```python
from build123d import *

# Parameters (mm, degrees)
BOSS_EXTRUDE1_DEPTH = 3
FILLET1_R           = 10
FILLET2_R           = 2
FILLET3_R           = 4
FILLET4_R           = 1
FILLET5_R           = 2
FILLET6_R           = 3
FILLET7_R           = 2
FILLET8_R           = 1


with BuildPart() as part:
    # Sketch1 → Boss-Extrude1 (new body)
    with BuildSketch(Plane(origin=(0, 0, 0), x_dir=(1, 0, 0), z_dir=(0, 1, 0))):
        with BuildLine():
            Line((0, 0), (0, 7.21))
            ThreePointArc((0, 7.21), (1.5, 8.71), (3, 7.21))
            Line((3, 7.21), (3, 0))
            ThreePointArc((3, 0), (10.063508451, 2.530649612), (15.2, 8))
            Line((15.2, 8), (20.9, 10.15))
            Line((20.9, 10.15), (22, 15.56))
            Line((22, 15.56), (30.53, 20))
            Line((30.53, 20), (21.94, 28))
            Line((21.94, 28), (18.834507406, 25.494802254))
            Line((18.834507406, 25.494802254), (22.601722061, 20.824888578))
            Line((22.601722061, 20.824888578), (16.53, 18.68))
            ThreePointArc((16.53, 18.68), (13.852574152, 13.870404311), (8.467766761, 12.728183128))
            Line((8.467766761, 12.728183128), (-3.6, 15.4))
            Line((-3.6, 15.4), (-6, 24.68))
            Line((-6, 24.68), (-7.84518958, 28))
            Line((-7.84518958, 28), (-8.88, 34.5))
            Line((-8.88, 34.5), (-2.152236064, 35.529882091))
            Line((-2.152236064, 35.529882091), (-2.387170471, 36.974018228))
            ThreePointArc((-2.387170471, 36.974018228), (-7.295622624, 39.289989721), (-12.7222653, 39.199569746))
            Line((-12.7222653, 39.199569746), (-14.412236064, 37.968616292))
            Line((-14.412236064, 37.968616292), (-12.083283256, 30.98175787))
            Line((-12.083283256, 30.98175787), (-11.160586433, 20.989038892))
            Line((-11.160586433, 20.989038892), (-7.18770511, 13.356453829))
            ThreePointArc((-7.18770511, 13.356453829), (-7.478060289, 11.939326713), (-8.633960614, 11.06958547))
            Line((-8.633960614, 11.06958547), (-15.174962181, 15.236636279))
            Line((-15.174962181, 15.236636279), (-18.788682966, 16.406314301))
            Line((-18.788682966, 16.406314301), (-23.978484738, 20.454374352))
            Line((-23.978484738, 20.454374352), (-19.760487577, 25.795906403))
            Line((-19.760487577, 25.795906403), (-20.917206202, 26.691855832))
            ThreePointArc((-20.917206202, 26.691855832), (-26.082048226, 24.977316424), (-29.953541863, 21.152819654))
            Line((-29.953541863, 21.152819654), (-30.35, 19.1))
            Line((-30.35, 19.1), (-23.881685757, 15.578477225))
            Line((-23.881685757, 15.578477225), (-16.391850065, 8.899542932))
            Line((-16.391850065, 8.899542932), (-4.31, 0))
            Line((-4.31, 0), (0, 0))
        make_face()
    extrude(amount=BOSS_EXTRUDE1_DEPTH)

    # Fillet1
    # the kernel refuses this fillet: 10 mm, written as the material it adds along each edge
    with BuildSketch(Plane(origin=(-23.881685757, 0, -15.578477225), x_dir=(0.7463543086555258, 0, 0.6655488306287767), z_dir=(0, 1, 0))) as fillet1_piece_1:
        with BuildLine():
            CenterArc((FILLET1_R * 0.115344853594, -FILLET1_R), FILLET1_R, 90, 13.159392789)
            Line((-FILLET1_R * 0.112315955105, -FILLET1_R * 0.0262595026484), (0, 0))
            Line((0, 0), (FILLET1_R * 0.115344853594, 0))
        make_face()
    extrude(amount=3)
    with BuildSketch(Plane(origin=(-18.788682966, 0, -16.406314301), x_dir=(0.9514034075145552, 0, 0.3079473269403278), z_dir=(0, 1, 0))) as fillet1_piece_2:
        with BuildLine():
            CenterArc((FILLET1_R * 0.176495798458, FILLET1_R), FILLET1_R, 249.981238779, 20.018761221)
            Line((-FILLET1_R * 0.165832024258, FILLET1_R * 0.0604194224044), (0, 0))
            Line((0, 0), (FILLET1_R * 0.176495798458, 0))
        make_face()
    extrude(amount=3)
    with BuildSketch(Plane(origin=(-12.083283256, 0, -30.98175787), x_dir=(-0.3162277660168379, 0, -0.9486832980505138), z_dir=(0, 1, 0))) as fillet1_piece_3:
        with BuildLine():
            CenterArc((FILLET1_R * 0.115344853594, FILLET1_R), FILLET1_R, 256.840607211, 13.159392789)
            Line((-FILLET1_R * 0.112315955105, FILLET1_R * 0.0262595026484), (0, 0))
            Line((0, 0), (FILLET1_R * 0.115344853594, 0))
        make_face()
    extrude(amount=3)
    # the kernel refuses this fillet: 10 mm, written as the material it takes off along each edge
    with BuildSketch(Plane(origin=(-16.391850065, -1.167802292, -8.899542932), x_dir=(-0.7463543086555279, 0, -0.6655488306287745), z_dir=(0, 1, 0))) as fillet1_2_piece_1:
        with BuildLine():
            CenterArc((FILLET1_R * 0.0467120916838, -FILLET1_R), FILLET1_R, 90, 5.348923188)
            Line((-FILLET1_R * 0.0465086821366, -FILLET1_R * 0.00435453733353), (0, 0))
            Line((0, 0), (FILLET1_R * 0.0467120916838, 0))
        make_face()
    extrude(amount=5.335604584, mode=Mode.SUBTRACT)
    with BuildSketch(Plane(origin=(-11.160586433, -4.90982012, -20.989038892), x_dir=(-0.09194577532432974, 0, -0.9957640154173116), z_dir=(0, 1, 0))) as fillet1_2_piece_2:
        with BuildLine():
            CenterArc((FILLET1_R * 0.196392804796, -FILLET1_R), FILLET1_R, 90, 22.222134755)
            Line((-FILLET1_R * 0.18180564018, -FILLET1_R * 0.0742754533783), (0, 0))
            Line((0, 0), (FILLET1_R * 0.196392804796, 0))
        make_face()
    extrude(amount=12.81964024, mode=Mode.SUBTRACT)
    with BuildSketch(Plane(origin=(-6, -3.194649605, -24.68), x_dir=(0.2503828219685178, 0, 0.9681469116116013), z_dir=(0, 1, 0))) as fillet1_2_piece_3:
        with BuildLine():
            CenterArc((FILLET1_R * 0.127785984198, -FILLET1_R), FILLET1_R, 90, 14.564262893)
            Line((-FILLET1_R * 0.123679735642, -FILLET1_R * 0.0321337945019), (0, 0))
            Line((0, 0), (FILLET1_R * 0.127785984198, 0))
        make_face()
    extrude(amount=9.38929921, mode=Mode.SUBTRACT)

    # Fillet2
    fillet2_edges = [part.edges().sort_by_distance(p)[0] for p in [
        (-30.35, 1.5, -19.1),
        (-14.412236064, 1.5, -37.968616292),
    ]]
    fillet(fillet2_edges, radius=FILLET2_R)

    # Fillet3
    # the kernel refuses this fillet: 4 mm, written as the material it takes off along each edge
    with BuildSketch(Plane(origin=(-12.7222653, -2.572689519, -39.199569746), x_dir=(-0.8083072770831305, 0, 0.5887608562179175), z_dir=(0, 1, 0))) as fillet3_piece_1:
        with BuildLine():
            CenterArc((0.875361271, 3.992337402), FILLET3_R, 243.063834504, 23.389134387)
            ThreePointArc((-0.936628841, 0.426290314), (-0.472898898, 0.203072318), (0, 0))
            Line((0, 0), (0.627889929, 0))
        make_face()
    extrude(amount=8.145379038, mode=Mode.SUBTRACT)
    with BuildSketch(Plane(origin=(-29.953541863, -2.496436383, -21.152819654), x_dir=(-0.18962458073088623, 0, 0.9818566689607173), z_dir=(0, 1, 0))) as fillet3_piece_2:
        with BuildLine():
            CenterArc((0.842574318, 3.994234672), FILLET3_R, 243.941405888, 22.981988472)
            ThreePointArc((-0.914585995, 0.400853585), (-0.461476033, 0.190882795), (0, 0))
            Line((0, 0), (0.627889929, 0))
        make_face()
    extrude(amount=7.992872766, mode=Mode.SUBTRACT)

    # Fillet4
    fillet4_edges = [part.edges().sort_by_distance(p)[0] for p in [
        (-20.917206202, 1.5, -26.691855832),
        (-19.760487577, 1.5, -25.795906403),
        (-2.387170471, 1.5, -36.974018228),
        (-2.152236064, 1.5, -35.529882091),
    ]]
    fillet(fillet4_edges, radius=FILLET4_R)

    # Fillet5
    fillet5_edges = [part.edges().sort_by_distance(p)[0] for p in [
        (-23.978484738, 1.5, -20.454374352),
        (-8.88, 1.5, -34.5),
    ]]
    fillet(fillet5_edges, radius=FILLET5_R)

    # Fillet6
    fillet6_edges = [part.edges().sort_by_distance(p)[0] for p in [
        (-4.31, 1.5, 0),
        (-3.6, 1.5, -15.4),
        (30.53, 1.5, -20),
        (22, 1.5, -15.56),
        (20.9, 1.5, -10.15),
        (15.2, 1.5, -8),
    ]]
    fillet(fillet6_edges, radius=FILLET6_R)

    # Fillet7
    fillet7_edges = [part.edges().sort_by_distance(p)[0] for p in [
        (16.53, 1.5, -18.68),
        (21.94, 1.5, -28),
    ]]
    fillet(fillet7_edges, radius=FILLET7_R)

    # Fillet8
    fillet8_edges = [part.edges().sort_by_distance(p)[0] for p in [
        (22.601722061, 1.5, -20.824888578),
        (18.834507406, 1.5, -25.494802254),
    ]]
    fillet(fillet8_edges, radius=FILLET8_R)


solid = part.part
```
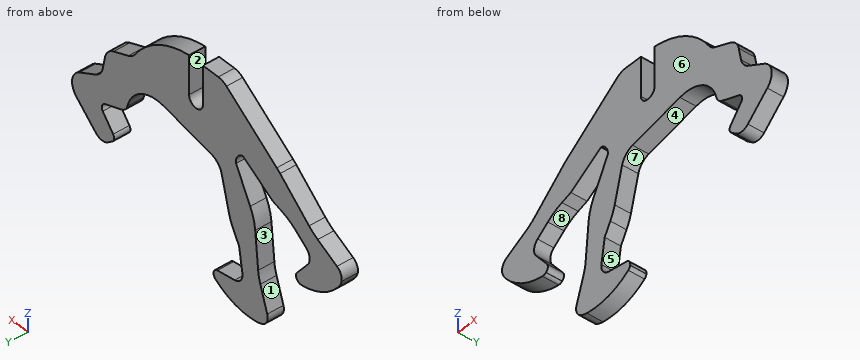
The model under review builds one solid part; all positions refer to its coordinate system, in mm. Face numbers are marked on the shaded views. A direction names the side the tool comes from. Give positions to 0.01 mm unless a question says otherwise; leave off trailing zeros. Order: outer loops, then holes, each group sorted by start corner. A loop starts at its lowest first (then second) coordinate and runs counter-clockwise, first axis right, second up. Notation, with made-up numbers: (-26, 2) - (10, 2) arc R20 ccw to (10, 41) - close; hole circle Ø6 at (-31.5, 32). An arc over 180 degrees is marked (long way). Use CSV: the item, a comma, the result in double quotes. Start each with the question number.
Q1. We need section A-A, the plane x = 14. Write out the cut boundary in (y, z), and give its area (3 significant figures).
Q2. Clearance check with a flat-ended pin moving along its axis: pin 1 Ø1 at (y, z) = (1, -25) entering from +X. State where the tip first meets the part, or that it passes through.
Q3. The part is to be moulded in two halves that separate along Z. For the marked faces 6, 7 and 8, say which applies: +Z half, -Z half, draft (parallel to the pull), parting line (faces both ways), or undercut.
Q4. To check wall thickness, follow line 1 along X through (y, z) = (2.4, -21); line 2 along X through (y, z) = (2.4, -24) (3 decimals); line 3 along X through (y, z) = (0.5, -5). State the ranges of each line that lie inside material, in increasing order. Write a range as [from, to].
Q5. We need section B-B, the plane x = 5. Write out the cut boundary in (y, z), and give its area (3 significant figures).
Q6. Tool access review of the marked faces 1, 2, 3, 4 and 5: name each direction out of +Z, -Z, +X, -X, +Y, -Y from which nothing blocks a thin tool from reaching the whole face with its end or side.
Outcome:
1,outline,"(0, -13.98) - (3, -13.98) - (3, -6.19) - (0, -6.19) - close"
1,area,"23.4 mm^2"
2,pin 1,"stops at x = 25.7"
3,face 6,"draft"
3,face 7,"undercut"
3,face 8,"-Z half"
4,line 1,"x = [-29.93, -23.15], [-10.96, -5.05], [21.89, 28.36]"
4,line 2,"x = [-27.45, -21.179], [-11.439, -5.842], [20.04, 26.235]"
4,line 3,"x = [-11.1, 0], [3, 12.99]"
5,outline,"(0, -13.5) - (3, -13.5) - (3, -0.35) - (0, -0.35) - close"
5,area,"39.5 mm^2"
6,face 1,"-X, +Y, -Y"
6,face 2,"+Z, +Y, -Y"
6,face 3,"+Y, -Y"
6,face 4,"-Z, +Y, -Y"
6,face 5,"+X, +Y, -Y"
